Geometry check sheet. Reference: the model listing, model coordinates, mm. Face numbers are marked on the shaded views. A direction names the side the tool comes from. Coordinates: 2 decimals unless noted, no trailing zeros. Loops run counter-clockwise (first coordinate to the right, second up) from the corner with the lowest first, then second, coordinate; pieces in that order, holes last. Notation, with made-up numbers: (78.5, 89) - (133.5, 89) arc R21 ccw to (133.5, 126) - close; hole circle Ø1 at (36.5, 78.5). An arc over 180 degrees is marked (long way). Write item = value, one per line. Start each with the question number.
Autodesk Inventor part; units mm, degrees
ref_plane "Work Plane1" through (33.575, 0, 0) normal (0, 0, -1) x (1, 0, 0)
ref_plane "YZ Plane" through (0, 0, 0) normal (1, 0, 0) x (0, 1, 0)
ref_plane "XZ Plane" through (0, 0, 0) normal (0, 1, 0) x (-1, 0, 0)
sketch "Sketch1" plane through (0, 0, 0) normal (0, 0, 1) x (1, 0, 0)
  line L0 (0, 0) -> (19.05, 0)
  line L1 (19.05, 0) -> (19.05, 3.175)
  line L2 (19.05, 3.175) -> (6.731, 3.175)
  line L3 (6.731, 3.175) -> (5.461, 3.175)
  line L4 (5.461, 3.175) -> (3.556, 3.175)
  line L5 (3.556, 3.175) -> (0.6048, 5.7404)
  line L6 (0.6048, 5.7404) -> (0, 5.7404)
  line L7 (0, 5.7404) -> (0, 0)
  line L8 (6.731, 3.175) -> (3.556, 3.175) construction
  line L9 (-3.81, 0) -> (22.86, 0)
  line L10 (0, 6.8885) -> (0, -1.1481)
  dimension "d0" = 19.05
  dimension "d1" = 41
  dimension "d2" = 1.27
  dimension "d3" = 12.319
  dimension "d4" = 3.556
  dimension "d5" = 6.35
  dimension "d6" = 6.35
  dimension "d7" = 11.4808
revolve "Body" add sketch "Sketch1" angle 360 about axis through (0, 0, 0) along (1, 0, 0)
sketch "Sketch2" plane through (0, 0, 0) normal (-1, 0, 0) x (0, 0, 1)
  line L0 (5.7404, -0.9525) -> (-5.7404, -0.9525)
  line L1 (-5.7404, -0.9525) -> (-5.7404, 0.9525)
  line L2 (-5.7404, 0.9525) -> (5.7404, 0.9525)
  line L3 (5.7404, 0.9525) -> (5.7404, -0.9525)
  line L4 (0, 0.9525) -> (0, -0.9525) construction
  line L5 (-5.7404, 0) -> (5.7404, 0) construction
  line L6 (0, 5.7404) -> (0, 0)
  dimension "d15" = 1.905
  dimension "d16" = 11.4808
extrude "Slot" cut sketch "Sketch2" against normal blind 1.7272
thread "Thread"
chamfer "Chamfer1" distance 0.7556 distance2 0.635 1 edges at (19.05, -3.175, 0) measured on face at (19.05, 0.3445, 0.7363)
fillet "Radius" radius 2.54 1 edges at (3.556, -3.175, 0)
ref_plane "Work Plane1" through (33.575, 0, 0) normal (0, 0, -1) x (1, 0, 0)
equation "\"d0\" = NLG"
equation "\"d1\" = 0.5 * SEWI"
equation "\"d2\" = GAL"
equation "\"d3\" = GEL"
equation "\"d4\" = KOH"
equation "\"d5\" = BDM"
equation "\"d6\" = GD"
equation "\"d7\" = KOD"
equation "\"d15\" = SBR"
equation "\"d16\" = KOD"
equation "\"d8\" = STI"
equation "\"d41\" = RR"
equation "\"d10\" = GEL"
equation "\"d12\" = -0.5 * SPD + 0.5 * GD"
equation "\"d13\" = 0.5 * GAL"
equation "\"NLG\" = 19.05"
equation "\"GAL\" = 1.27"
equation "\"GEL\" = 12.319"
equation "\"KOH\" = 3.556"
equation "\"KOD\" = 11.4808"
equation "\"SEWI\" = 82deg"
equation "\"BDM\" = NND"
equation "\"GD\" = NND"
equation "\"SBR\" = 1.905"
equation "\"STI\" = 1.7272"
equation "\"SPD\" = 4.8387"
equation "\"RR\" = 2.54"
equation "\"GUL\" = 0.75565"
equation "\"TOA\" = 30deg"
equation "\"THREADDIA\" = 6.35"
equation "\"HHPTC\" = 1.27"
equation "\"NND\" = 6.35"
equation "\"GD1\" = SPD"
properties part number "ANSI B18.6.2 - 1/4-20 UNC x 0.75" material "Steel, Mild"
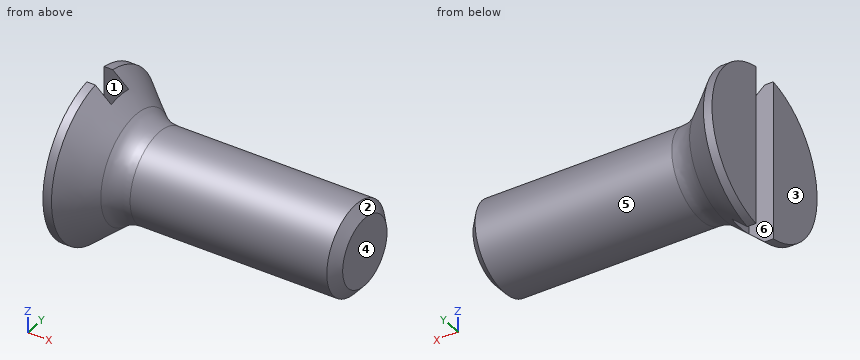
(1) Tool access check on the marked faces 4, 5 and 6. Record the directions out of +Z, -Z, +X, -X, +Y, -Y that give a thin tool (end or side, any length) a straight path to the whole face; none if there is none.
(2) Scan lines: line 1 (X direction, y = -0.75, z = -2.25); line 2 (Y direction, x = 11.25, z = 0) (3 decimals); line 3 (Y direction, x = 5.25, z = 1). Record each from-to range of solid material in increasing order.
(3) Depth check by flat-ended pin: pin 1 (1 mm diameter, centred on x = 4, y = 2, fed in from +Z); pin 2 (3 mm diameter, centred on x = 10, y = 2.5, fed in from +Z); pin 3 (6 mm diameter, centred on x = 12, y = -2, fed in from -Z) (3 decimals); pin 4 (1 mm diameter, centred on x = 7, y = 4, fed in from +Z). Enter the tip coordinate at first touch or a pass-through.
(4) Draft check along Y on the marked faces 1, 2 and 3. Enter one of: pulls with the +Y half, pulls with the -Y half, needs draft (parallel to the pull), parting line crosses it, or undercut.
(5) Sectioned sample at A-A on x = 5.25. Enter the section's corners in (y, z) (3 decimals), plus the area to 3 significant figures.
Working result:
q1.face_4 = +Z, -Z, +X, +Y, -Y
q1.face_5 = +X
q1.face_6 = +Z, -Z, -X
q2.line_1 = 1.73 to 19.05
q2.line_2 = -3.175 to 3.175
q2.line_3 = -3.01 to 3.01
q3.pin_1 = 2.89
q3.pin_2 = 3.01
q3.pin_3 = -3.175
q3.pin_4 = through
q4.face_1 = undercut
q4.face_2 = parting line crosses it
q4.face_3 = needs draft
q5.outline = circle Ø6.35 at (0, 0)
q5.area = 31.7 mm2
